Geometry check sheet. Reference: the model listing, model coordinates, mm. A direction names the side the tool comes from. Round coordinates to 2 decimals unless told otherwise and drop trailing zeros. Order: outer loops, then holes, each group sorted by start corner. A loop starts at its lowest first (then second) coordinate and runs counter-clockwise, first axis right, second up. Notation, with made-up numbers: (23, 2) -> (49, 2) arc R23 cw to (49, 41) -> close; hole circle Ø2 at (-30, 69). An arc over 180 degrees is marked (long way). Use a Markdown table: item, result. Add a question column.
Item 1: Sectioned sample at C-C, the plane x = -29. Record the cut outline in (y, z).
Item 2: Set-up check for faces 5 (the flat face through (-48, 3, 23)), 6 (the flat face through (101, 3, 21.291)), 7 (the flat face through (95, 3, -22)): record each of +Z, -Z, +X, -X, +Y, -Y from which the full face is reachable in a straight line by a thin tool's end or side.
Item 3: Sectioned sample at B-B, the plane z = -20.5. Record the cut outline in (x, y).
Item 4: Material ranges on probe 1 along X at (y, z) = (3.25, 25); probe 2 along X at (y, z) = (1.9, 17); probe 3 along X at (y, z) = (2.1, 17.5), recorded low to high. Write a range as [from, to].
Item 5: Gauge pin test, flat ends, axial feed: pin 1 Ø2 at (x, y) = (83.5, 3.5) entering from +Z; pin 2 Ø0.5 at (y, z) = (4.5, 6) entering from +X; pin 3 Ø1 at (y, z) = (4.5, 9) entering from -X. Record the tip position at first contact, or that the pin passes through.
Item 6: Mould release check, pull along Z, two halves, no side actions. Record for faces 1 (the flat face through (-65, 3, 29)), 2 (the flat face through (34.5, 3, 26)), 3 (the flat face through (-91, 3, 2.519)), 4 (the flat face through (15, 3, -26)): pulls with the +Z half, pulls with the -Z half, needs draft (parallel to the pull), parting line crosses it, or undercut.
Item 7: Sectioned sample at A-A, the plane x = -4.5. Record the cut outline in (y, z).
from build123d import *

# Parameters (mm, degrees)
SKETCH_1_W      = 30
SKETCH_1_H      = 6
EXTRUDE_1_DEPTH = 6


with BuildPart() as part:
    # Эскиз1 → Бобышка-Вытянуть1 (new body)
    with BuildSketch(Plane(origin=(0, 0, 0), x_dir=(1, 0, 0), z_dir=(0, 1, 0))):
        Polygon((-95, 23), (-95, 13.709265489), (-107, 13.709265489), (-107, 3.709265489), (-95, 3.709265489), (-95, -2.518957871), (-86.2, -2.518957871), (-86.2, -0.901182203), (-84, -0.901182203), (-84, -2.518957871), (-82, -2.518957871), (-82, -5.062511151), (-84, -5.062511151), (-84, -6.68028682), (-86.2, -6.68028682), (-86.2, -5.062511151), (-95, -5.062511151), (-95, -11.290734511), (-107, -11.290734511), (-107, -21.290734511), (-95, -21.290734511), (-95, -23), (-69.5, -23), (-69.5, -29), (-59.5, -29), (-59.5, -23), (-53.4, -23), (-53.4, -17.2), (-54.9, -17.2), (-54.9, -15), (-53.4, -15), (-53.4, -13), (-50.6, -13), (-50.6, -15), (-49.1, -15), (-49.1, -17.2), (-50.6, -17.2), (-50.6, -23), (-44.5, -23), (-44.5, -29), (-34.5, -29), (-34.5, -23), (34.5, -23), (34.5, -29), (44.5, -29), (44.5, -23), (50.6, -23), (50.6, -17.2), (49.1, -17.2), (49.1, -15), (50.6, -15), (50.6, -13), (53.4, -13), (53.4, -15), (54.9, -15), (54.9, -17.2), (53.4, -17.2), (53.4, -23), (59.5, -23), (59.5, -29), (69.5, -29), (69.5, -23), (95, -23), (95, -21.290734511), (107, -21.290734511), (107, -11.290734511), (95, -11.290734511), (95, -5.062511151), (86.2, -5.062511151), (86.2, -6.68028682), (84, -6.68028682), (84, -5.062511151), (82, -5.062511151), (82, -2.518957871), (84, -2.518957871), (84, -0.901182203), (86.2, -0.901182203), (86.2, -2.518957871), (95, -2.518957871), (95, 3.709265489), (107, 3.709265489), (107, 13.709265489), (95, 13.709265489), (95, 23), (95, 31), (-95, 31), align=None)
        with Locations((0, 26)):
            Rectangle(SKETCH_1_W, SKETCH_1_H, mode=Mode.SUBTRACT)
    extrude(amount=EXTRUDE_1_DEPTH)


solid = part.part
Found:
| question | item | result |
|---|---|---|
| 1 | outline | (0, -31) -> (6, -31) -> (6, 23) -> (0, 23) -> close |
| 2 | face 5 | +Z, +Y, -Y |
| 2 | face 6 | +Z, +X, +Y, -Y |
| 2 | face 7 | -Z, +X, +Y, -Y |
| 3 | outline | (-95, 0) -> (95, 0) -> (95, 6) -> (-95, 6) -> close |
| 4 | probe 1 | x = [-69.5, -59.5], [-44.5, -34.5], [34.5, 44.5], [59.5, 69.5] |
| 4 | probe 2 | x = [-107, -54.9], [-49.1, 49.1], [54.9, 107] |
| 4 | probe 3 | x = [-107, -53.4], [-50.6, 50.6], [53.4, 107] |
| 5 | pin 1 | stops at z = 23 |
| 5 | pin 2 | stops at x = 95 |
| 5 | pin 3 | stops at x = -95 |
| 6 | face 1 | pulls with the +Z half |
| 6 | face 2 | needs draft |
| 6 | face 3 | undercut |
| 6 | face 4 | undercut |
| 7 | outline | (0, -31) -> (6, -31) -> (6, -29) -> (0, -29) -> close; (0, -23) -> (6, -23) -> (6, 23) -> (0, 23) -> close |
